Model file for the job. Use its own axes, mm. A direction names the side the tool comes from. Round coordinates to 2 decimals unless told otherwise and drop trailing zeros. Put each result on its own line as item: value. Start each with the question number.
Q1. Flat gauge pins, fed straight in: P1, Ø2.5, axis at y = 76.825, z = -9.525, coming from the +X side (3 decimals); P2, Ø0.8, axis at y = 76.5, z = -10, coming from the -X side (3 decimals). Where does each tip first touch, or does it go through?
Q2. Pull direction Z, two halves, no side cores. Call faces 1 (the face through (9.525, 77, -10)), 2 (the face through (47, 80, -38)), 3 (the face through (47, 77, 0)), 4 (the face through (4.696, 77.965, -8.798)): released by +Z, released by -Z, zero draft, split by the parting line, or undercut.
Q3. 3-axis set-ups, long thin cutter, end or side, ignore diameter. For faces 5 (the face through (86.475, 77, -10)), 6 (the face through (47, 73.65, -38)), 7 (the face through (9.525, 77, -65)): which of +Z, -Z, +X, -X, +Y, -Y reach the whole face in a straight line?
from build123d import *

# Parameters (mm, degrees)
SKETCH1_W           = 96
SKETCH1_H           = 75
BOSS_EXTRUDE1_DEPTH = 6.35
SKETCH2_R           = 1.35255
CUT_EXTRUDE1_DEPTH  = 9.525
SKETCH3_R           = 1.35255
CUT_EXTRUDE2_DEPTH  = 9.525


with BuildPart() as part:
    # Sketch1 → Boss-Extrude1 (new body)
    with BuildSketch(Plane(origin=(0, 80, 0), x_dir=(1, 0, 0), z_dir=(0, 1, 0))):
        with Locations((48, 37.5)):
            Rectangle(SKETCH1_W, SKETCH1_H)
    extrude(amount=-BOSS_EXTRUDE1_DEPTH)

    # Sketch2 → Cut-Extrude1 (cut)
    with BuildSketch(Plane(origin=(96, 0, 0), x_dir=(0, 0, -1), z_dir=(1, 0, 0))):
        with Locations((65.475, 76.825)):
            Circle(SKETCH2_R)
        with Locations((9.525, 76.825)):
            Circle(SKETCH2_R)
    extrude(amount=-CUT_EXTRUDE1_DEPTH, mode=Mode.SUBTRACT)

    # Sketch3 → Cut-Extrude2 (cut)
    with BuildSketch(Plane.ZY):
        with Locations((-65.475, 76.825)):
            Circle(SKETCH3_R)
        with Locations((-9.525, 76.825)):
            Circle(SKETCH3_R)
    extrude(amount=-CUT_EXTRUDE2_DEPTH, mode=Mode.SUBTRACT)


solid = part.part
Ans:
1. P1: stops at x = 86.475
1. P2: stops at x = 9.525
2. face 1: undercut
2. face 2: zero draft
2. face 3: released by +Z
2. face 4: undercut
3. face 5: +X
3. face 6: +Z, -Z, +X, -X, -Y
3. face 7: -X
